The model under review builds one solid part; all positions refer to its coordinate system, in mm. A direction names the side the tool comes from. Coordinates: 2 decimals unless noted, no trailing zeros. Answer in a Markdown table with one row per item.
```python
from build123d import *
from build123d.topology import SkipClean

# Parameters (mm, degrees)
BOSS_EXTRUDE1_DEPTH     = 8
CUT_EXTRUDE1_DEPTH      = 78.289612463
CUT_EXTRUDE1_DEPTH_BACK = 70.289612463
CUT_EXTRUDE1_START      = -8
SKETCH9_R               = 5
CUT_EXTRUDE2_DEPTH      = 70.289612463
CUT_EXTRUDE2_DEPTH_BACK = 70.289612463
CUT_EXTRUDE3_DEPTH      = 70.289612463
CUT_EXTRUDE3_DEPTH_BACK = 70.289612463
SKETCH11_R              = 15.5
CUT_EXTRUDE4_DEPTH      = 70.289612463
CUT_EXTRUDE4_DEPTH_BACK = 70.289612463
SKETCH12_W              = 5.7
SKETCH12_H              = 2.4
CUT_EXTRUDE5_START      = 28.174078
CUT_EXTRUDE5_DEPTH      = 6
CHAMFER1_SIZE           = 2
MOVE_START              = -8
MOVE_FACE1_OUTLINE_W    = 59
MOVE_FACE1_OUTLINE_H    = 67
MOVE_FACE1_DEPTH        = 0.1
MOVE_START_2            = 7.9
MOVE_FACE1_2_OUTLINE_W  = 59
MOVE_FACE1_2_OUTLINE_H  = 67
MOVE_FACE1_2_DEPTH      = 0.1


# Read off the part's stored shape, not the designer's step: Move Face1
with BuildPart() as part:
    # Sketch2 → Boss-Extrude1 (new, symmetric)
    with BuildSketch(Plane.YZ):
        with BuildLine():
            Line((-12.727922061, -32.553844327), (-14.317300295, -30.964466094))
            ThreePointArc((-14.317300295, -30.964466094), (-15.939417039, -29.880602337), (-17.852834201, -29.5))
            Line((-17.852834201, -29.5), (-28, -29.5))
            ThreePointArc((-28, -29.5), (-48.859650045, -20.859650045), (-57.5, 0))
            Line((-57.5, 0), (-57.5, 28.174077734))
            Line((-57.5, 28.174077734), (0, 28.174077734))
            Line((0, 28.174077734), (0, -37.825922266))
            ThreePointArc((0, -37.825922266), (-6.888301783, -36.455753851), (-12.727922061, -32.553844327))
        make_face()
    extrude(amount=BOSS_EXTRUDE1_DEPTH, both=True)

    # Sketch9 → Cut-Extrude1 (cut, two sides: drawn at the far end of the back side and taken through both)
    with BuildSketch(Plane.YZ.offset(CUT_EXTRUDE1_START - CUT_EXTRUDE1_DEPTH_BACK)):
        with Locations((0, 4.174077734)):
            Circle(SKETCH9_R)
        with Locations((0, -19.825922266)):
            Circle(SKETCH9_R)
    extrude(amount=CUT_EXTRUDE1_DEPTH + CUT_EXTRUDE1_DEPTH_BACK, mode=Mode.SUBTRACT)

    # Sketch10 → Cut-Extrude2 (cut, two sides: drawn at the far end of the back side and taken through both)
    with BuildSketch(Plane.YZ.offset(-CUT_EXTRUDE2_DEPTH_BACK)):
        Polygon((2.078460969, 12.574077734), (4.156921938, 16.174077734), (2.078460969, 19.774077734), (-2.078460969, 19.774077734), (-4.156921938, 16.174077734), (-2.078460969, 12.574077734), align=None)
        Polygon((-5.545893683, -31.250591332), (-4.470003116, -27.235313074), (-7.409390808, -24.295925382), (-11.424669066, -25.371815949), (-12.500559632, -29.387094207), (-9.561171941, -32.326481898), align=None)
        Polygon((4.156921938, -31.825922266), (2.078460969, -28.225922266), (-2.078460969, -28.225922266), (-4.156921938, -31.825922266), (-2.078460969, -35.425922266), (2.078460969, -35.425922266), align=None)
        Polygon((12.500559632, -29.387094207), (11.424669066, -25.371815949), (7.409390808, -24.295925382), (4.470003116, -27.235313074), (5.545893683, -31.250591332), (9.561171941, -32.326481898), align=None)
        Polygon((-51, 17.517155796), (-47.4, 19.595616765), (-47.4, 23.752538703), (-51, 25.830999672), (-54.6, 23.752538703), (-54.6, 19.595616765), align=None)
    extrude(amount=CUT_EXTRUDE2_DEPTH + CUT_EXTRUDE2_DEPTH_BACK, mode=Mode.SUBTRACT)

    # Sketch11 → Cut-Extrude3 (cut, two sides: drawn at the far end of the back side and taken through both)
    with BuildSketch(Plane.YZ.offset(-CUT_EXTRUDE3_DEPTH_BACK)):
        with Locations(Location((-28, 0, 0), (0, 0, 270))):
            Circle(SKETCH11_R)
    extrude(amount=CUT_EXTRUDE3_DEPTH + CUT_EXTRUDE3_DEPTH_BACK, mode=Mode.SUBTRACT)

    # Sketch12 → Cut-Extrude4 (cut, two sides: drawn at the far end of the back side and taken through both)
    with BuildSketch(Plane.YZ.offset(-CUT_EXTRUDE4_DEPTH_BACK)):
        with Locations((-40, 24.974077734)):
            Rectangle(SKETCH12_W, SKETCH12_H)
        with Locations((0, 24.974077734)):
            Rectangle(SKETCH12_W, SKETCH12_H)
    extrude(amount=CUT_EXTRUDE4_DEPTH + CUT_EXTRUDE4_DEPTH_BACK, mode=Mode.SUBTRACT)

    # Sketch13 → Cut-Extrude5 (cut)
    with BuildSketch(Plane.XY.offset(CUT_EXTRUDE5_START)):
        Polygon((0, -2.404163056), (2.404163056, 0), (0, 2.404163056), (-2.404163056, 0), align=None)
        Polygon((0, -42.404163056), (2.404163056, -40), (0, -37.595836944), (-2.404163056, -40), align=None)
    extrude(amount=-CUT_EXTRUDE5_DEPTH, mode=Mode.SUBTRACT)

    # Chamfer1
    chamfer1_edges = [part.edges().sort_by_distance(p)[0] for p in [
        (8, -22.9264171, -29.5),
        (8, -48.859650045, -20.859650045),
        (8, -57.5, 14.087038867),
        (-8, -48.859650045, -20.859650045),
        (-8, -28, 15.5),
        (8, -28, 15.5),
        (-8, -22.9264171, -29.5),
        (-8, -15.939417039, -29.880602337),
        (-8, -13.522611178, -31.759155211),
        (-8, -6.888301783, -36.455753851),
        (-8, -57.5, 14.087038867),
        (8, -6.888301783, -36.455753851),
        (8, -13.522611178, -31.759155211),
        (8, -15.939417039, -29.880602337),
    ]]
    chamfer(chamfer1_edges, length=CHAMFER1_SIZE)

    # Move Face1 outline → Move Face1 (cut)
    with BuildSketch(Plane.YZ.offset(MOVE_START)):
        with Locations((-27.5, -3.5)):
            Rectangle(MOVE_FACE1_OUTLINE_W, MOVE_FACE1_OUTLINE_H)
    extrude(amount=MOVE_FACE1_DEPTH, mode=Mode.SUBTRACT)

    # Move Face1 2 outline → Move Face1 2 (cut)
    with BuildSketch(Plane.YZ.offset(MOVE_START_2)):
        with Locations((-27.5, -3.5)):
            Rectangle(MOVE_FACE1_2_OUTLINE_W, MOVE_FACE1_2_OUTLINE_H)
    extrude(amount=MOVE_FACE1_2_DEPTH, mode=Mode.SUBTRACT)

    # Mirror1: part across plane


with BuildPart() as part_1:
    with SkipClean():  # the faces are left unmerged after this step: merging them gives an invalid solid
        add(part.part)
        add(part.part.mirror(Plane(origin=(0, 0, 0), x_dir=(0, 0, 1), z_dir=(0, -1, 0))))


solid = part_1.part
```
Item 1: We need section A-A, the plane z = -3. State how many separate pieces and enclosed holes the cut face has, then the cut area to 3 significant figures.
Check values:
| item | result |
|---|---|
| separate pieces | 3 |
| enclosed holes | 0 |
| area | 829 mm^2 |
Item 2: To check wall thickness, follow line 1 (Y direction, x = 3.25, z = 25); line 2 (Y direction, x = 1, z = -7); line 3 (Z direction, x = 4.5, y = -3). State the ranges of each line that lie inside material, in increasing order. Write a range as from..to.
Check values:
| item | result |
|---|---|
| line 1 | -57.5..-52.44, -49.56..-42.85, -37.15..-2.85, 2.85..37.15, 42.85..49.56, 52.44..57.5 |
| line 2 | -56.66..-41.83, -14.17..14.17, 41.83..56.66 |
| line 3 | -37.57..-33.83, -29.82..-23.83, -15.83..0.17, 8.17..14.17, 18.18..28.17 |
Item 3: Clearance check with flat-ended pins moving along their axes: pin 1 Ø8 at (x, z) = (3, -8) entering from -Y; pin 2 Ø5 at (x, y) = (-1, -24.5) entering from -Z; pin 3 Ø5 at (x, z) = (-1, -16.5) entering from -Y; pin 4 Ø9 at (y, z) = (0, 4.17) entering from -X. State where each tip first meets the part, or that it passes through.
Check values:
| item | result |
|---|---|
| pin 1 | y = -57.23 |
| pin 2 | z = -29.5 |
| pin 3 | y = -53.97 |
| pin 4 | through |
Item 4: Tool access review of faces 1 (the face through (0, 57.5, 14)), 2 (the face through (0, 2.85, 25)), 3 (the face through (1.185, 41.219, 22.985)): name each direction out of +Z, -Z, +X, -X, +Y, -Y from which nothing blocks a thin tool from reaching the whole face with its end or side.
Check values:
| item | result |
|---|---|
| face 1 | +Z, -Z, +X, -X, +Y |
| face 2 | +X, -X |
| face 3 | +Z |
Item 5: Mouldability with a two-part tool opening along Z and no side actions: class faces 4 (the face through (1.185, -41.219, 22.985)), 5 (the face through (2, 1, 28.174)), 6 (the face through (-0.111, 9.389, -24.826)) as +Z half, -Z half, draft (parallel to the pull), parting line (faces both ways), or undercut.
Check values:
| item | result |
|---|---|
| face 4 | draft |
| face 5 | +Z half |
| face 6 | undercut |
